from build123d import *

# Parameters (mm, degrees)
BOSS_EXTRUDE1_DEPTH     = 1
CUT_EXTRUDE1_DEPTH      = 71.717748833
CUT_EXTRUDE1_DEPTH_BACK = 71.717748833
SKETCH2_R               = 2


with BuildPart() as part:
    # Sketch1 → Boss-Extrude1 (new body)
    with BuildSketch(Plane(origin=(0, 0, 0), x_dir=(1, 0, 0), z_dir=(0, 1, 0))):
        Polygon((17.5, 50), (32.5, 50), (32.5, 15), (50, 15), (50, 0), (0, 0), (0, 15), (17.5, 15), align=None)
    extrude(amount=BOSS_EXTRUDE1_DEPTH)

    # Sketch2 → Cut-Extrude1 (cut, two sides: drawn at the far end of the back side and taken through both)
    with BuildSketch(Plane(origin=(0, 1, 0), x_dir=(1, 0, 0), z_dir=(0, 1, 0)).offset(-CUT_EXTRUDE1_DEPTH_BACK)):
        with Locations(Location((41.25, 7.5, 0), (0, 0, 270))):
            Circle(SKETCH2_R)
        with Locations(Location((25, 40.5, 0), (0, 0, 270))):
            Circle(SKETCH2_R)
        with Locations(Location((25, 24, 0), (0, 0, 270))):
            Circle(SKETCH2_R)
        with Locations(Location((8.75, 7.5, 0), (0, 0, 270))):
            Circle(SKETCH2_R)
    extrude(amount=CUT_EXTRUDE1_DEPTH + CUT_EXTRUDE1_DEPTH_BACK, mode=Mode.SUBTRACT)


solid = part.part
Source: CAD feature listing. Evaluate the final solid. Frame: model axes, mm. Coordinates: 2 decimals unless noted, no trailing zeros. Write each loop counter-clockwise with the first axis right and the second up, starting at its lowest first coordinate (ties: lowest second). Pieces come first, ordered by that corner, then holes. Notation, with made-up numbers: M 19.25,47.25 L 29.25,47.25 A10 cw 29.25,66.25 Z; hole C -4.75,-3.75 d9. An arc over 180 degrees is marked long. Use a Markdown table: item, result.
1) Section B-B, the plane y = 0.2. Output: boundary loops of the cut face in (x, z), then the cut area to 3 significant figures.
Conclusion:
| item | result |
|---|---|
| outline | M 0,-15 L 17.5,-15 L 17.5,-50 L 32.5,-50 L 32.5,-15 L 50,-15 L 50,0 L 0,0 Z; hole C 8.75,-7.5 d4; hole C 25,-40.5 d4; hole C 25,-24 d4; hole C 41.25,-7.5 d4 |
| area | 1,220 mm^2 |
2) Section C-C, the plane x = 8.75. Output: boundary loops of the cut face in (y, z), then the cut area to 3 significant figures.
Conclusion:
| item | result |
|---|---|
| outline | M 0,-15 L 1,-15 L 1,-9.5 L 0,-9.5 Z; M 0,-5.5 L 1,-5.5 L 1,0 L 0,0 Z |
| area | 11.0 mm^2 |
3) Section A-A, the plane z = -24. Output: boundary loops of the cut face in (x, y).
Conclusion:
| item | result |
|---|---|
| outline | M 17.5,0 L 23,0 L 23,1 L 17.5,1 Z; M 27,0 L 32.5,0 L 32.5,1 L 27,1 Z |
4) Mould query, pull axis X, two halves, no side actions, for faces 1 (the flat face through (25, 0, -20)), 2 (the cylindrical face through (23.8, 0.5, -25.6)), 3 (the cylindrical face through (39.298, 0.493, -7.934)). Classes: pulls with the +X half, pulls with the -X half, needs draft (parallel to the pull), parting line crosses it, or undercut.
Conclusion:
| item | result |
|---|---|
| face 1 | needs draft |
| face 2 | undercut |
| face 3 | undercut |
5) Section D-D, the plane x = 25. Output: boundary loops of the cut face in (y, z).
Conclusion:
| item | result |
|---|---|
| outline | M 0,-50 L 1,-50 L 1,-42.5 L 0,-42.5 Z; M 0,-38.5 L 1,-38.5 L 1,-26 L 0,-26 Z; M 0,-22 L 1,-22 L 1,0 L 0,0 Z |
6) Ray query, L1, parallel to Z at x = 25, y = 0.2; L2, parallel to X at y = 0.2, z = -7.5; L3, parallel to Z at x = 41.25, y = 0.35. Return the intervals inside material, ascending.
Conclusion:
| item | result |
|---|---|
| L1 | z = -50 to -42.5, -38.5 to -26, -22 to 0 |
| L2 | x = 0 to 6.75, 10.75 to 39.25, 43.25 to 50 |
| L3 | z = -15 to -9.5, -5.5 to 0 |
